Geometry check sheet. Reference: the model listing, model coordinates, mm. A direction names the side the tool comes from. Coordinates: 2 decimals unless noted, no trailing zeros. Order: outer loops, then holes, each group sorted by start corner. A loop starts at its lowest first (then second) coordinate and runs counter-clockwise, first axis right, second up. Notation, with made-up numbers: (56, 30.5) - (84, 30.5) arc R35 ccw to (84, 64.5) - close; hole circle Ø3 at (73.5, 51.5). An arc over 180 degrees is marked (long way). Return JSON: item names as keys, results as strings. Group by question number.
Item 1: Section check B-B on z = 2.75. Enter the section's corners in (x, y).
Item 2: Scan lines: probe 1 along X at (y, z) = (-2.5, 6.5); probe 2 along X at (y, z) = (-1, 1); probe 3 along Y at (x, z) = (22.5, 5). Record each from-to range of solid material in increasing order.
Item 3: Section check D-D on y = 2.5. Enter the section's corners in (x, z).
Item 4: Draft check along Y on faces 1 (the flat face through (30, 3, 4)), 2 (the flat face through (24, -1, 2)), 3 (the flat face through (19, 7.25, 5)). Enter one of: pulls with the +Y half, pulls with the -Y half, needs draft (parallel to the pull), parting line crosses it, or undercut.
Item 5: Tool access check on faces 4 (the flat face through (14, 4, 7.8)), 5 (the flat face through (4, -3, 7.9)), 6 (the flat face through (7.7, -3, 7)), 7 (the cylindrical face through (3.2, 0, 7.9)). Record the directions out of +Z, -Z, +X, -X, +Y, -Y that give a thin tool (end or side, any length) a straight path to the whole face; none if there is none.
Item 6: Section check A-A on y = -2.5. Enter the section's corners in (x, z), then the cut area to 3 significant figures.
Item 7: Gauge pin test, flat ends, axial feed: pin 1 (1.3 mm diameter, centred on x = 3.5, y = -2, fed in from +Z); pin 2 (5 mm diameter, centred on x = 15, z = 2, fed in from +Y). Record the tip position at first contact, or that the pin passes through.
Item 8: Section check C-C on x = 16. Enter the section's corners in (y, z), then the cut area to 3 significant figures.
Autodesk Fusion 360 part; units mm, degrees
sketch "Boceto1" plane through (0, 0, 0) normal (0, 0, 1) x (1, 0, 0)
  line L0 (0, 7.25) -> (30, 7.25)
  line L1 (30, 7.25) -> (30, -4.25)
  line L2 (30, -4.25) -> (0, -4.25)
  line L3 (0, -4.25) -> (0, 7.25)
  dimension "d1" = 30
  dimension "d2" = 11.5
  dimension "d3" = 7.25
extrude "Extruir1" add sketch "Boceto1" along normal blind 2
sketch "Boceto2" plane through (0, 0, 2) normal (0, 0, 1) x (-1, 0, 0)
  line L0 (0, 4.25) -> (-30, 4.25)
  line L1 (-30, 4.25) -> (-30, -7.25)
  line L2 (-30, -7.25) -> (0, -7.25)
  line L3 (0, -7.25) -> (0, 4.25)
  line L4 (0, -1.23) -> (-30, -1.23)
  line L5 (0, 1.23) -> (-30, 1.23)
  line L6 (-6.35, -1.23) -> (-6.35, 1.23)
  line L7 (-9.2, -1.23) -> (-9.2, 1.23)
  line L8 (-18, -1.23) -> (-18, 1.23)
  line L9 (0, -0.5) -> (-30, -0.5)
  dimension "d6" = 2.46
  dimension "d7" = 1.23
  dimension "d8" = 6.35
  dimension "d9" = 9.2
  dimension "d10" = 18
extrude "Extruir2" add sketch "Boceto2" along normal blind 5.9 contours L3 L5 L6 L9 | L3 L4 L6 L9
sketch "Boceto3" plane through (0, -1.23, 0) normal (0, -1, 0) x (1, 0, 0)
  line L0 (0, 2) -> (6.35, 2)
  line L1 (6.35, 2) -> (6.35, 7.9)
  line L2 (6.35, 7.9) -> (0, 7.9)
  line L3 (0, 7.9) -> (0, 2)
  arc A0 (6.35, 4.725) -> (0, 4.725) centre (3.175, 4.725) ccw
  point P0 (3.175, 4.725)
  dimension "d13" = 3.175
  dimension "d14" = 3.175
  dimension "d54" = 3.175
  dimension "d55" = 3.175
extrude "Extruir3" cut sketch "Boceto3" against normal blind 3 contours L2 L3 A0 | L1 L2 A0
extrude "Extruir4" cut sketch "Boceto2" against normal blind 2 contours L5 L7 L8 L9 | L4 L7 L8 L9
extrude "Extruir5" add sketch "Boceto2" along normal blind 5.9 contours L0 L1 L3 L5 | L1 L2 L3 L4
chamfer "Chaflán1" distance 1.8 angle 45 2 edges at (7.775, 1.23, 2) (24, 1.23, 2)
sketch "Boceto4" plane through (0, -1.23, 0) normal (0, 1, 0) x (-1, 0, 0)
  line L0 (-18, 2) -> (-18, 0)
  line L1 (-18, 0) -> (-9.2, 0)
  line L2 (-9.2, 0) -> (-9.2, 2)
  line L3 (-9.2, 2) -> (-6.35, 2)
  line L4 (-6.35, 2) -> (-6.35, 4.725)
  arc A0 (-3.175, 7.9) -> (-6.35, 4.725) centre (-3.175, 4.725) ccw
  line L5 (-3.175, 7.9) -> (-30, 7.9)
  line L6 (-30, 7.9) -> (-30, 2)
  line L7 (-30, 2) -> (-18, 2)
  line L8 (-9.2, 2) -> (-18, 2)
extrude "Extruir6" cut sketch "Boceto4" against normal blind 5 contours L0 L1 L2 L8
sketch "Boceto5" plane through (0, 1.23, 0) normal (0, -1, 0) x (1, 0, 0)
  line L0 (9.2, 3.8) -> (9.2, 0)
  line L1 (9.2, 0) -> (18, 0)
  line L2 (18, 0) -> (18, 3.8)
  line L3 (30, 3.8) -> (30, 7.9)
  line L4 (30, 7.9) -> (3.175, 7.9)
  arc A0 (6.35, 4.725) -> (3.175, 7.9) centre (3.175, 4.725) ccw
  line L5 (6.35, 4.725) -> (6.35, 3.8)
  line L6 (18, 3.8) -> (9.2, 3.8)
  line L7 (18, 3.8) -> (30, 3.8)
  line L8 (6.35, 3.8) -> (9.2, 3.8)
extrude "Extruir7" cut sketch "Boceto5" against normal blind 7 contours L0 L1 L2 L6
extrude "Extruir8" cut 2 faces at (15.0667, -2.2367, 2) (12.1333, 5.2433, 3.8) along direction (0, 0, 1) blind 4
extrude "Extruir10" add 1 faces at (11.0583, 5.2433, 7.9) along direction (0, 0, 1) blind 2.5
sketch "Boceto8" plane through (0, 0, 7.9) normal (0, 0, 1) x (-1, 0, 0)
  line L0 (-3.175, 1.23) -> (0, 1.23)
  line L1 (0, 1.23) -> (0, 4.25)
  line L2 (0, 4.25) -> (-30, 4.25)
  line L3 (-30, 4.25) -> (-30, 1.23)
  line L4 (-30, 1.23) -> (-3.175, 1.23)
  line L5 (-7.7, 1.23) -> (-7.7, 4.25)
  line L6 (-20.5, 1.23) -> (-20.5, 4.25)
  point P0 (0, 4.25)
  point P1 (-9.2, 4.25)
  point P2 (-18, 4.25)
  point P3 (-30, 4.25)
  dimension "d41" = 9.2
  dimension "d42" = 7.7
  dimension "d43" = 12
  dimension "d44" = 9.5
extrude "Extruir12" cut sketch "Boceto8" against normal blind 2 contours L2 L4 L5 L6
fillet "Empalme4" radius 0.5 29 edges at (0, -2.74, 7.9) (3.85, -4.25, 7.9) (7.7, -2.74, 7.9) (7.7, -4.25, 6.9) (7.7, -1.23, 6.9) (7.7, -2.74, 5.9) (8.45, -1.23, 5.9) (8.45, -4.25, 5.9) (9.2, -2.74, 5.9) (19.25, -1.23, 5.9) (18, -2.74, 5.9) (19.25, -4.25, 5.9) (20.5, -2.74, 7.9) (25.25, -1.23, 7.9) (25.25, -4.25, 7.9) (20.5, -1.23, 6.9) (20.5, -4.25, 6.9) (20.5, -2.74, 5.9) (15, 1.23, 10.4) (0, 4.24, 10.4) (30, 4.24, 10.4) (0, -4.25, 3.95) (9.2, -4.25, 2.95) (18, -4.25, 2.95) (30, -4.25, 3.95) (0, 1.23, 7.5625) (30, 1.23, 7.1) (30, -1.23, 4.95) (0, -1.23, 6.3125)
fillet "Empalme5" radius 0.8 2 edges at (9.2, 4.24, 7.8) (18, 4.24, 7.8)
equation "d3 = d2 / 2 + 1.5 mm"
equation "d7 = d6 / 2"
equation "d9 = d10 - 8.8 mm"
equation "d13 = d8 / 2"
equation "d14 = d13"
equation "d42 = d41 - 1.5 mm"
equation "d44 = d43 - 2.5 mm"
equation "d54 = d8 / 2"
equation "d55 = d8 / 2"
Computed:
{
 "1": {"outline": "(0, -3.75) arc R0.5 ccw to (0.5, -4.25) - (8.7, -4.25) arc R0.5 ccw to (9.2, -3.75) - (9.2, -1.23) - (6.35, -1.23) - (6.35, 0.18) - (9.2, 0.18) - (9.2, 7.25) - (0, 7.25) - close; (18, -3.75) arc R0.5 ccw to (18.5, -4.25) - (29.5, -4.25) arc R0.5 ccw to (30, -3.75) - (30, -1.73) arc R0.5 ccw to (29.5, -1.23) - (18, -1.23) - close; (18, 0.18) - (30, 0.18) - (30, 7.25) - (18, 7.25) - close"},
 "2": {"probe 1": "x = 0 to 7.7, 20.5 to 30", "probe 2": "x = 0 to 9.2, 18 to 30", "probe 3": "y = -4.25 to -1.23, 1.23 to 7.25"},
 "3": {"outline": "(0, 0) - (9.2, 0) - (9.2, 7) arc R0.8 cw to (10, 7.8) - (17.2, 7.8) arc R0.8 cw to (18, 7) - (18, 0) - (30, 0) - (30, 9.9) arc R0.5 ccw to (29.5, 10.4) - (0.5, 10.4) arc R0.5 ccw to (0, 9.9) - close"},
 "4": {"face 1": "needs draft", "face 2": "undercut", "face 3": "pulls with the +Y half"},
 "5": {"face 4": "-Z, +Y, -Y", "face 5": "+Z, +X, -X, -Y", "face 6": "+Z, -Y", "face 7": "+Z"},
 "6": {"outline": "(0, 0) - (9.2, 0) - (9.2, 5.4) arc R0.5 ccw to (8.7, 5.9) - (8.2, 5.9) arc R0.5 cw to (7.7, 6.4) - (7.7, 7.4) arc R0.5 ccw to (7.2, 7.9) - (0.5, 7.9) arc R0.5 ccw to (0, 7.4) - close; (18, 0) - (30, 0) - (30, 7.9) - (21, 7.9) arc R0.5 ccw to (20.5, 7.4) - (20.5, 6.4) arc R0.5 cw to (20, 5.9) - (18.5, 5.9) arc R0.5 ccw to (18, 5.4) - close", "area": "159 mm²"},
 "7": {"pin 1": "stops at z = 7.9", "pin 2": "passes through"},
 "8": {"outline": "(1.23, 7.8) - (7.25, 7.8) - (7.25, 10.4) - (1.73, 10.4) arc R0.5 ccw to (1.23, 9.9) - close", "area": "15.6 mm²"}
}
